Here's how the part is built. I have some questions about the finished solid (model axes, mm). Face numbers are marked on the shaded views. A direction names the side the tool comes from. Round coordinates to 2 decimals unless told otherwise and drop trailing zeros. Loops run counter-clockwise (first coordinate to the right, second up) from the corner with the lowest first, then second, coordinate; pieces in that order, holes last. Notation, with made-up numbers: M 28.5,83 L 80.5,83 A29 ccw 80.5,118 Z; hole C 28,84.25 d6. An arc over 180 degrees is marked long. Use a Markdown table: item, result.
```python
from build123d import *
from OCP.BRepFilletAPI import BRepFilletAPI_MakeChamfer

# Parameters (mm, degrees)
SKETCH1_W           = 6.858
SKETCH1_H           = 5.334
BOSS_EXTRUDE1_DEPTH = 6.35
SKETCH2_W           = 1.524
SKETCH2_H           = 1.524
BOSS_EXTRUDE2_DEPTH = 4.826
CHAMFER1_SIZE       = 0.9398
CHAMFER1_SIZE2      = 0.542593783
BOSS_EXTRUDE3_START = -3.048
SKETCH3_W           = 0.720393783
SKETCH3_H           = 1.524
SKETCH3_W_2         = 0.981406217
SKETCH3_W_3         = 1.524
SKETCH3_H_2         = 1.1176
SKETCH3_H_3         = 0.5842
SKETCH3_H_4         = 0.981406217
SKETCH3_H_5         = 0.720393783
BOSS_EXTRUDE3_DEPTH = 0.2032
SKETCH4_W           = 1.397
SKETCH4_H           = 1.524
SKETCH4_W_2         = 1.524
SKETCH4_H_2         = 1.397
CUT_EXTRUDE1_DEPTH  = 3.556
SKETCH5_W           = 1.524
SKETCH5_H           = 1.143
BOSS_EXTRUDE4_DEPTH = 0.254
FILLET1_R           = 0.127
FILLET2_R           = 0.0508
FILLET3_R           = 0.635
FILLET4_R           = 0.254
FILLET5_R           = 0.254
FILLET6_R           = 1.27


with BuildPart() as part:
    # Sketch1 → Boss-Extrude1 (new body)
    with BuildSketch(Plane(origin=(0, 0, 0), x_dir=(1, 0, 0), z_dir=(0, 1, 0))):
        Rectangle(SKETCH1_W, SKETCH1_H)
    extrude(amount=BOSS_EXTRUDE1_DEPTH)

    # Sketch2 → Boss-Extrude2 (add)
    with BuildSketch(Plane(origin=(0, 6.35, 0), x_dir=(1, 0, 0), z_dir=(0, 1, 0))):
        Rectangle(SKETCH2_W, SKETCH2_H)
        with Locations((1.524, 0)):
            Rectangle(SKETCH2_W, SKETCH2_H)
        with Locations((0, 1.524)):
            Rectangle(SKETCH2_W, SKETCH2_H)
        with Locations((-1.524, 0)):
            Rectangle(SKETCH2_W, SKETCH2_H)
        with Locations((0, -1.524)):
            Rectangle(SKETCH2_W, SKETCH2_H)
    extrude(amount=BOSS_EXTRUDE2_DEPTH)

    # Chamfer1: one chamfer whose edges measure the first distance from different faces: ONE call of the kernel's chamfer builder (chamfer() names one face for all edges)
    chamfer1_edges_1 = [part.edges().sort_by_distance(p)[0] for p in [
        (2.286, 11.176, 0),
    ]]
    chamfer1_side_1 = [part.faces().sort_by_distance(p)[0] for p in [
        (2.286, 8.763, 0),
    ]]
    chamfer1_edges_2 = [part.edges().sort_by_distance(p)[0] for p in [
        (0, 11.176, -2.286),
    ]]
    chamfer1_side_2 = [part.faces().sort_by_distance(p)[0] for p in [
        (0, 11.176, 0),
    ]]
    chamfer1_edges_3 = [part.edges().sort_by_distance(p)[0] for p in [
        (-2.286, 11.176, 0),
    ]]
    chamfer1_side_3 = [part.faces().sort_by_distance(p)[0] for p in [
        (-2.286, 8.763, 0),
    ]]
    chamfer1_edges_4 = [part.edges().sort_by_distance(p)[0] for p in [
        (0, 11.176, 2.286),
    ]]
    chamfer1_side_4 = [part.faces().sort_by_distance(p)[0] for p in [
        (0, 8.763, 2.286),
    ]]
    chamfer1 = BRepFilletAPI_MakeChamfer(part.part.solid().wrapped)
    for e in chamfer1_edges_1:
        chamfer1.Add(CHAMFER1_SIZE, CHAMFER1_SIZE2, e.wrapped, chamfer1_side_1[0].wrapped)  # the first distance lies on this face
    for e in chamfer1_edges_2:
        chamfer1.Add(CHAMFER1_SIZE, CHAMFER1_SIZE2, e.wrapped, chamfer1_side_2[0].wrapped)  # the first distance lies on this face
    for e in chamfer1_edges_3:
        chamfer1.Add(CHAMFER1_SIZE, CHAMFER1_SIZE2, e.wrapped, chamfer1_side_3[0].wrapped)  # the first distance lies on this face
    for e in chamfer1_edges_4:
        chamfer1.Add(CHAMFER1_SIZE, CHAMFER1_SIZE2, e.wrapped, chamfer1_side_4[0].wrapped)  # the first distance lies on this face
    add(Compound.cast(chamfer1.Shape()), mode=Mode.REPLACE)

    # Sketch3 → Boss-Extrude3 (add)
    with BuildSketch(Plane(origin=(0, 11.176, 0), x_dir=(1, 0, 0), z_dir=(0, 1, 0)).offset(BOSS_EXTRUDE3_START)):
        with Locations((2.103603109, 0)):
            Rectangle(SKETCH3_W, SKETCH3_H)
        with Locations((1.252703108, 0)):
            Rectangle(SKETCH3_W_2, SKETCH3_H)
        with Locations((0, 1.905)):
            Rectangle(SKETCH3_W_3, SKETCH3_H_2)
        with Locations((0, 1.0541)):
            Rectangle(SKETCH3_W_3, SKETCH3_H_3)
        Rectangle(SKETCH3_W_3, SKETCH3_H)
        with Locations((-1.252703108, 0)):
            Rectangle(SKETCH3_W_2, SKETCH3_H)
        with Locations((-2.103603109, 0)):
            Rectangle(SKETCH3_W, SKETCH3_H)
        with Locations((0, -1.252703108)):
            Rectangle(SKETCH3_W_3, SKETCH3_H_4)
        with Locations((0, -2.103603109)):
            Rectangle(SKETCH3_W_3, SKETCH3_H_5)
    extrude(amount=BOSS_EXTRUDE3_DEPTH)

    # Sketch4 → Cut-Extrude1 (cut)
    with BuildSketch(Plane.XZ):
        with Locations((-1.4605, 0)):
            Rectangle(SKETCH4_W, SKETCH4_H)
        Rectangle(SKETCH4_W_2, SKETCH4_H)
        with Locations((1.4605, 0)):
            Rectangle(SKETCH4_W, SKETCH4_H)
        with Locations((0, -1.4605)):
            Rectangle(SKETCH4_W_2, SKETCH4_H_2)
        with Locations((0, 1.4605)):
            Rectangle(SKETCH4_W_2, SKETCH4_H_2)
    extrude(amount=-CUT_EXTRUDE1_DEPTH, mode=Mode.SUBTRACT)

    # Sketch5 → Boss-Extrude4 (add)
    with BuildSketch(Plane(origin=(0, 0, 2.159), x_dir=(-1, 0, 0), z_dir=(0, 0, -1))):
        with Locations((0, 2.3495)):
            Rectangle(SKETCH5_W, SKETCH5_H)
    extrude(amount=BOSS_EXTRUDE4_DEPTH)

    # Fillet1
    fillet1_edges = [part.edges().sort_by_distance(p)[0] for p in [
        (0, 1.778, 1.905),
        (0, 2.921, 1.905),
    ]]
    fillet(fillet1_edges, radius=FILLET1_R)

    # Fillet2
    fillet2_edges = [part.edges().sort_by_distance(p)[0] for p in [
        (-2.4638, 8.3312, 0),
        (0, 8.3312, 2.4638),
        (2.4638, 8.128, 0),
        (2.4638, 8.3312, 0),
        (2.4638, 8.2296, 0.762),
        (2.4638, 8.2296, -0.762),
        (0, 8.3312, -2.4638),
        (0.762, 8.2296, -2.4638),
        (-0.762, 8.2296, -2.4638),
        (-2.4638, 8.128, 0),
        (-2.4638, 8.2296, -0.762),
        (0, 8.128, 2.4638),
        (-0.762, 8.2296, 2.4638),
        (0, 8.128, -2.4638),
        (-2.4638, 8.2296, 0.762),
        (0.762, 8.2296, 2.4638),
    ]]
    fillet(fillet2_edges, radius=FILLET2_R)

    # Fillet3
    fillet3_edges = [part.edges().sort_by_distance(p)[0] for p in [
        (3.429, 3.175, 2.667),
        (-3.429, 3.175, -2.667),
        (3.429, 3.175, -2.667),
    ]]
    fillet(fillet3_edges, radius=FILLET3_R)

    # Fillet4
    fillet4_edges = [part.edges().sort_by_distance(p)[0] for p in [
        (-1.4605, 0, -0.762),
        (-2.159, 0, 0),
        (0.762, 0, 1.4605),
        (1.4605, 0, -0.762),
        (0.762, 0, -1.4605),
        (0, 0, -2.159),
        (-0.762, 0, -1.4605),
        (2.159, 0, 0),
        (1.4605, 0, 0.762),
        (0, 0, 2.159),
        (-0.762, 0, 1.4605),
        (-1.4605, 0, 0.762),
    ]]
    fillet(fillet4_edges, radius=FILLET4_R)

    # Fillet5
    # the kernel refuses this fillet: 0.254 mm, written as the material it takes off along each edge
    with BuildSketch(Plane(origin=(1.016, 0.254, -1.016), x_dir=(0, 0, 1), z_dir=(-1, 0, 0))) as fillet5_piece_1_section:
        Polygon((0, 0), (FILLET5_R, 0), (FILLET5_R, -FILLET5_R), (0, -FILLET5_R), align=None)
    fillet5_piece_1 = extrude(amount=FILLET5_R, mode=Mode.PRIVATE)
    fillet5_piece_1 = fillet5_piece_1 - Plane(origin=(1.016, 0.254, -1.016), x_dir=(0, 0.7071067811865475, -0.7071067811865475), z_dir=(-1, 0, 0)) * Sphere(FILLET5_R, mode=Mode.PRIVATE)
    add(fillet5_piece_1, mode=Mode.SUBTRACT)
    with BuildSketch(Plane(origin=(1.016, 0.254, 1.016), x_dir=(0, 0, -1), z_dir=(-1, 0, 0))) as fillet5_piece_2_section:
        Polygon((0, 0), (FILLET5_R, 0), (FILLET5_R, FILLET5_R), (0, FILLET5_R), align=None)
    fillet5_piece_2 = extrude(amount=FILLET5_R, mode=Mode.PRIVATE)
    fillet5_piece_2 = fillet5_piece_2 - Plane(origin=(1.016, 0.254, 1.016), x_dir=(0, 0.7071067811865475, 0.7071067811865475), z_dir=(-1, 0, 0)) * Sphere(FILLET5_R, mode=Mode.PRIVATE)
    add(fillet5_piece_2, mode=Mode.SUBTRACT)
    with BuildSketch(Plane(origin=(-1.016, 0.254, -1.016), x_dir=(1, 0, 0), z_dir=(0, 0, 1))) as fillet5_piece_3_section:
        Polygon((0, 0), (FILLET5_R, 0), (FILLET5_R, -FILLET5_R), (0, -FILLET5_R), align=None)
    fillet5_piece_3 = extrude(amount=FILLET5_R, mode=Mode.PRIVATE)
    fillet5_piece_3 = fillet5_piece_3 - Plane(origin=(-1.016, 0.254, -1.016), x_dir=(-0.7071067811865475, 0.7071067811865475, 0), z_dir=(0, 0, 1)) * Sphere(FILLET5_R, mode=Mode.PRIVATE)
    add(fillet5_piece_3, mode=Mode.SUBTRACT)
    with BuildSketch(Plane(origin=(-1.016, 0.254, 1.016), x_dir=(1, 0, 0), z_dir=(0, 0, -1))) as fillet5_piece_4_section:
        Polygon((0, 0), (FILLET5_R, 0), (FILLET5_R, FILLET5_R), (0, FILLET5_R), align=None)
    fillet5_piece_4 = extrude(amount=FILLET5_R, mode=Mode.PRIVATE)
    fillet5_piece_4 = fillet5_piece_4 - Plane(origin=(-1.016, 0.254, 1.016), x_dir=(-0.7071067811865475, 0.7071067811865475, 0), z_dir=(0, 0, -1)) * Sphere(FILLET5_R, mode=Mode.PRIVATE)
    add(fillet5_piece_4, mode=Mode.SUBTRACT)
    with BuildSketch(Plane(origin=(-0.762, 0.254, -0.762), x_dir=(-1, 0, 0), z_dir=(0, 1, 0)), Plane(origin=(0.762, 0.254, -0.762), x_dir=(0, 0, -1), z_dir=(0, 1, 0))) as fillet5_piece_5:
        with BuildLine():
            CenterArc((FILLET5_R, -FILLET5_R), FILLET5_R, 90, 90)
            Line((0, -FILLET5_R), (0, 0))
            Line((0, 0), (FILLET5_R, 0))
        make_face()
    extrude(amount=3.302, mode=Mode.SUBTRACT)
    with BuildSketch(Plane(origin=(-0.762, 0.254, 0.762), x_dir=(-1, 0, 0), z_dir=(0, 1, 0)), Plane(origin=(0.762, 0.254, 0.762), x_dir=(0, 0, 1), z_dir=(0, 1, 0))) as fillet5_piece_6:
        with BuildLine():
            CenterArc((FILLET5_R, FILLET5_R), FILLET5_R, 180, 90)
            Line((0, FILLET5_R), (0, 0))
            Line((0, 0), (FILLET5_R, 0))
        make_face()
    extrude(amount=3.302, mode=Mode.SUBTRACT)

    # Fillet6
    fillet6_edges = [part.edges().sort_by_distance(p)[0] for p in [
        (-3.429, 3.175, 2.667),
    ]]
    fillet(fillet6_edges, radius=FILLET6_R)


solid = part.part
```
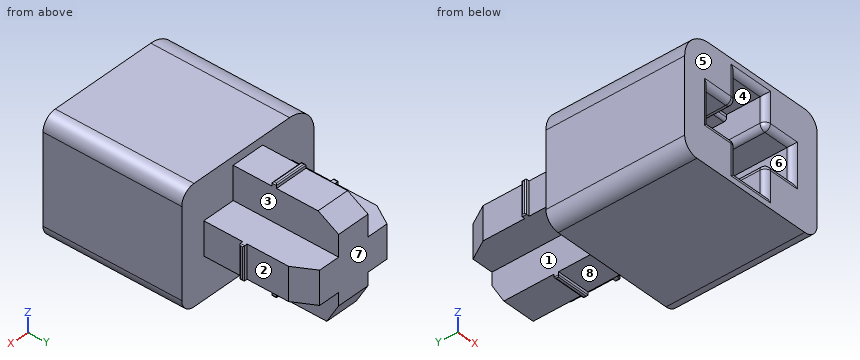
Q1. Will these pins go through, and if not, where does the flat tip stop? P1, Ø1.2, axis at y = 7, z = 0, coming from the +X side; P2, Ø3, axis at x = 0, y = 10, coming from the +Z side.
Return value:
| item | result |
|---|---|
| P1 | stops at x = 2.29 |
| P2 | stops at z = 2.29 |
Q2. Imagine slicing it at A-A, the plane z = -0.45. Please give me the cut outline in (x, y), then the cut area to 3 significant figures.
Return value:
| item | result |
|---|---|
| outline | M -3.43,0 L -2.41,0 A0.25 ccw -2.16,0.25 L -2.16,3.56 L 2.16,3.56 L 2.16,0.25 A0.25 ccw 2.41,0 L 3.43,0 L 3.43,6.35 L 2.29,6.35 L 2.29,8.13 L 2.41,8.13 A0.05 ccw 2.46,8.18 L 2.46,8.28 A0.05 ccw 2.41,8.33 L 2.29,8.33 L 2.29,10.24 L 1.74,11.18 L -1.74,11.18 L -2.29,10.24 L -2.29,8.33 L -2.41,8.33 A0.05 ccw -2.46,8.28 L -2.46,8.18 A0.05 ccw -2.41,8.13 L -2.29,8.13 L -2.29,6.35 L -3.43,6.35 Z |
| area | 49.8 mm^2 |
Q3. Imagine slicing it at D-D, the plane y = 9.75. Please give me the cut outline in (x, z), then the cut area to 3 significant figures.
Return value:
| item | result |
|---|---|
| outline | M -2.29,-0.76 L -0.76,-0.76 L -0.76,-2.29 L 0.76,-2.29 L 0.76,-0.76 L 2.29,-0.76 L 2.29,0.76 L 0.76,0.76 L 0.76,2.29 L -0.76,2.29 L -0.76,0.76 L -2.29,0.76 Z |
| area | 11.6 mm^2 |
Q4. We'd pull the mould along Y, two halves only. Please class the marked faces 5, 6, 7 and 8: pulls with the +Y half, pulls with the -Y half, needs draft (parallel to the pull), parting line crosses it, or undercut.
Return value:
| item | result |
|---|---|
| face 5 | pulls with the -Y half |
| face 6 | needs draft |
| face 7 | pulls with the +Y half |
| face 8 | undercut |
Q5. For the marked faces 1, 2, 3 and 4, which set-ups out of +Z, -Z, +X, -X, +Y, -Y let a thin tool reach every point of the face, with its end or its side?
Return value:
| item | result |
|---|---|
| face 1 | -Z, -X, +Y |
| face 2 | +Z, -Z, +X, +Y |
| face 3 | +Z, +X, +Y |
| face 4 | -Y |
Q6. Imagine slicing it at B-B, the plane y = 3.25. Please give me the cut outline in (x, z) (3 decimals), then the cut area to 3 significant figures.
Return value:
| item | result |
|---|---|
| outline | M -3.429,-2.032 A0.635 ccw -2.794,-2.667 L 2.794,-2.667 A0.635 ccw 3.429,-2.032 L 3.429,2.032 A0.635 ccw 2.794,2.667 L -2.159,2.667 A1.27 ccw -3.429,1.397 Z; hole M -2.159,-0.762 L -1.016,-0.762 A0.254 cw -0.762,-1.016 L -0.762,-2.159 L 0.762,-2.159 L 0.762,-1.016 A0.254 cw 1.016,-0.762 L 2.159,-0.762 L 2.159,0.762 L 1.016,0.762 A0.254 cw 0.762,1.016 L 0.762,2.159 L -0.762,2.159 L -0.762,1.016 A0.254 cw -1.016,0.762 L -2.159,0.762 Z |
| area | 25.1 mm^2 |
Q7. I need wall thicknesses on line 1 (Z direction, x = 2, y = 3.5); line 2 (X direction, y = 2.5, z = -1.05); line 3 (X direction, y = 1.5, z = 0.15). Which ranges of each line are inside material? Lowest first, please. Write a range as from..to.
Return value:
| item | result |
|---|---|
| line 1 | z = -2.67..-0.76, 0.76..2.67 |
| line 2 | x = -3.43..-0.76, 0.76..3.43 |
| line 3 | x = -3.43..-2.16, 2.16..3.43 |
